from build123d import *

# Parameters (mm, degrees)
F1_W     = 1
F1_H     = 1
F1_W_2   = 13
F2_DEPTH = 0.5


with BuildPart() as f2:
    # F1 (on Top) → F2 (new body)
    with BuildSketch(Plane.XY):
        with BuildLine():
            ThreePointArc((38, -47.5), (37.7071067812, -46.7928932188), (37, -46.5))
            Line((37, -46.5), (37, -47.5))
            Line((37, -47.5), (36, -47.5))
            ThreePointArc((36, -47.5), (36.2928932188, -48.2071067812), (37, -48.5))
            ThreePointArc((37, -48.5), (37.7071067812, -48.2071067812), (38, -47.5))
        make_face()
        with BuildLine():
            Line((36, -46.5), (37, -46.5))
            ThreePointArc((37, -46.5), (37.7071067812, -46.7928932188), (38, -47.5))
            Line((38, -47.5), (38, 47.5))
            ThreePointArc((38, 47.5), (37, 48.5), (36, 47.5))
            Line((36, 47.5), (36, -46.5))
        make_face()
        with Locations((36.5, -47)):
            Rectangle(F1_W, F1_H)
        with Locations((29.5, -47)):
            Rectangle(F1_W_2, F1_H)
        with BuildLine():
            ThreePointArc((37, -48.5), (36.2928932188, -48.2071067812), (36, -47.5))
            Line((36, -47.5), (23, -47.5))
            ThreePointArc((23, -47.5), (22.7071067812, -48.2071067812), (22, -48.5))
            Line((22, -48.5), (37, -48.5))
        make_face()
        with BuildLine():
            Line((22, -46.5), (23, -46.5))
            Line((23, -46.5), (23, 47.5))
            ThreePointArc((23, 47.5), (22.7071067812, 46.7928932188), (22, 46.5))
            Line((22, 46.5), (22, -46.5))
        make_face()
        with Locations((22.5, -47)):
            Rectangle(F1_W, F1_H)
        with BuildLine():
            ThreePointArc((22, -48.5), (22.7071067812, -48.2071067812), (23, -47.5))
            Line((23, -47.5), (22, -47.5))
            Line((22, -47.5), (22, -46.5))
            ThreePointArc((22, -46.5), (21.2928932188, -46.7928932188), (21, -47.5))
            ThreePointArc((21, -47.5), (21.2928932188, -48.2071067812), (22, -48.5))
        make_face()
        with BuildLine():
            ThreePointArc((22, 46.5), (22.7071067812, 46.7928932188), (23, 47.5))
            ThreePointArc((23, 47.5), (22.7071067812, 48.2071067812), (22, 48.5))
            ThreePointArc((22, 48.5), (21.2928932188, 48.2071067812), (21, 47.5))
            Line((21, 47.5), (22, 47.5))
            Line((22, 47.5), (22, 46.5))
        make_face()
        with BuildLine():
            ThreePointArc((21, -47.5), (21.2928932188, -46.7928932188), (22, -46.5))
            Line((22, -46.5), (22, 46.5))
            Line((22, 46.5), (21, 46.5))
            Line((21, 46.5), (21, -47.5))
        make_face()
        with BuildLine():
            ThreePointArc((21, 47.5), (21.2928932188, 48.2071067812), (22, 48.5))
            Line((22, 48.5), (7, 48.5))
            ThreePointArc((7, 48.5), (7.7071067812, 48.2071067812), (8, 47.5))
            Line((8, 47.5), (21, 47.5))
        make_face()
        with Locations((21.5, 47)):
            Rectangle(F1_W, F1_H)
        with Locations((14.5, 47)):
            Rectangle(F1_W_2, F1_H)
        with BuildLine():
            ThreePointArc((8, 47.5), (7.7071067812, 48.2071067812), (7, 48.5))
            ThreePointArc((7, 48.5), (6.2928932188, 48.2071067812), (6, 47.5))
            ThreePointArc((6, 47.5), (6.2928932188, 46.7928932188), (7, 46.5))
            Line((7, 46.5), (7, 47.5))
            Line((7, 47.5), (8, 47.5))
        make_face()
        with BuildLine():
            Line((8, -47.5), (8, 46.5))
            Line((8, 46.5), (7, 46.5))
            Line((7, 46.5), (7, -46.5))
            ThreePointArc((7, -46.5), (7.7071067812, -46.7928932188), (8, -47.5))
        make_face()
        with Locations((7.5, 47)):
            Rectangle(F1_W, F1_H)
        with BuildLine():
            ThreePointArc((7, 46.5), (6.2928932188, 46.7928932188), (6, 47.5))
            Line((6, 47.5), (6, -46.5))
            Line((6, -46.5), (7, -46.5))
            Line((7, -46.5), (7, 46.5))
        make_face()
        with BuildLine():
            ThreePointArc((7, -48.5), (7.7071067812, -48.2071067812), (8, -47.5))
            ThreePointArc((8, -47.5), (7.7071067812, -46.7928932188), (7, -46.5))
            Line((7, -46.5), (7, -47.5))
            Line((7, -47.5), (6, -47.5))
            ThreePointArc((6, -47.5), (6.2928932188, -48.2071067812), (7, -48.5))
        make_face()
        with Locations((6.5, -47)):
            Rectangle(F1_W, F1_H)
        with Locations((-0.5, -47)):
            Rectangle(F1_W_2, F1_H)
        with BuildLine():
            Line((-8, -48.5), (7, -48.5))
            ThreePointArc((7, -48.5), (6.2928932188, -48.2071067812), (6, -47.5))
            Line((6, -47.5), (-7, -47.5))
            ThreePointArc((-7, -47.5), (-7.2928932188, -48.2071067812), (-8, -48.5))
        make_face()
        with Locations((-7.5, -47)):
            Rectangle(F1_W, F1_H)
        with BuildLine():
            Line((-8, -46.5), (-7, -46.5))
            Line((-7, -46.5), (-7, 47.5))
            ThreePointArc((-7, 47.5), (-7.2928932188, 46.7928932188), (-8, 46.5))
            Line((-8, 46.5), (-8, -46.5))
        make_face()
        with BuildLine():
            ThreePointArc((-9, -47.5), (-8.7071067812, -48.2071067812), (-8, -48.5))
            ThreePointArc((-8, -48.5), (-7.2928932188, -48.2071067812), (-7, -47.5))
            Line((-7, -47.5), (-8, -47.5))
            Line((-8, -47.5), (-8, -46.5))
            ThreePointArc((-8, -46.5), (-8.7071067812, -46.7928932188), (-9, -47.5))
        make_face()
        with BuildLine():
            ThreePointArc((-9, -47.5), (-8.7071067812, -46.7928932188), (-8, -46.5))
            Line((-8, -46.5), (-8, 46.5))
            Line((-8, 46.5), (-9, 46.5))
            Line((-9, 46.5), (-9, -47.5))
        make_face()
        with BuildLine():
            ThreePointArc((-8, 46.5), (-7.2928932188, 46.7928932188), (-7, 47.5))
            ThreePointArc((-7, 47.5), (-7.2928932188, 48.2071067812), (-8, 48.5))
            ThreePointArc((-8, 48.5), (-8.7071067812, 48.2071067812), (-9, 47.5))
            Line((-9, 47.5), (-8, 47.5))
            Line((-8, 47.5), (-8, 46.5))
        make_face()
        with Locations((-8.5, 47)):
            Rectangle(F1_W, F1_H)
        with BuildLine():
            ThreePointArc((-9, 47.5), (-8.7071067812, 48.2071067812), (-8, 48.5))
            Line((-8, 48.5), (-23, 48.5))
            ThreePointArc((-23, 48.5), (-22.2928932188, 48.2071067812), (-22, 47.5))
            Line((-22, 47.5), (-9, 47.5))
        make_face()
        with Locations((-15.5, 47)):
            Rectangle(F1_W_2, F1_H)
        with BuildLine():
            ThreePointArc((-22, 47.5), (-22.2928932188, 48.2071067812), (-23, 48.5))
            ThreePointArc((-23, 48.5), (-23.7071067812, 48.2071067812), (-24, 47.5))
            ThreePointArc((-24, 47.5), (-23.7071067812, 46.7928932188), (-23, 46.5))
            Line((-23, 46.5), (-23, 47.5))
            Line((-23, 47.5), (-22, 47.5))
        make_face()
        with Locations((-22.5, 47)):
            Rectangle(F1_W, F1_H)
        with BuildLine():
            Line((-22, -47.5), (-22, 46.5))
            Line((-22, 46.5), (-23, 46.5))
            Line((-23, 46.5), (-23, -46.5))
            ThreePointArc((-23, -46.5), (-22.2928932188, -46.7928932188), (-22, -47.5))
        make_face()
        with BuildLine():
            ThreePointArc((-23, 46.5), (-23.7071067812, 46.7928932188), (-24, 47.5))
            Line((-24, 47.5), (-24, -46.5))
            Line((-24, -46.5), (-23, -46.5))
            Line((-23, -46.5), (-23, 46.5))
        make_face()
        with BuildLine():
            ThreePointArc((-23, -48.5), (-22.2928932188, -48.2071067812), (-22, -47.5))
            ThreePointArc((-22, -47.5), (-22.2928932188, -46.7928932188), (-23, -46.5))
            Line((-23, -46.5), (-23, -47.5))
            Line((-23, -47.5), (-24, -47.5))
            ThreePointArc((-24, -47.5), (-23.7071067812, -48.2071067812), (-23, -48.5))
        make_face()
        with Locations((-30.5, -47)):
            Rectangle(F1_W_2, F1_H)
        with Locations((-23.5, -47)):
            Rectangle(F1_W, F1_H)
        with BuildLine():
            Line((-38, -48.5), (-23, -48.5))
            ThreePointArc((-23, -48.5), (-23.7071067812, -48.2071067812), (-24, -47.5))
            Line((-24, -47.5), (-37, -47.5))
            ThreePointArc((-37, -47.5), (-37.2928932188, -48.2071067812), (-38, -48.5))
        make_face()
        with BuildLine():
            Line((-38, -46.5), (-37, -46.5))
            Line((-37, -46.5), (-37, 47.5))
            ThreePointArc((-37, 47.5), (-38, 48.5), (-39, 47.5))
            Line((-39, 47.5), (-39, -47.5))
            ThreePointArc((-39, -47.5), (-38.7071067812, -46.7928932188), (-38, -46.5))
        make_face()
        with Locations((-37.5, -47)):
            Rectangle(F1_W, F1_H)
        with BuildLine():
            ThreePointArc((-39, -47.5), (-38.7071067812, -48.2071067812), (-38, -48.5))
            ThreePointArc((-38, -48.5), (-37.2928932188, -48.2071067812), (-37, -47.5))
            Line((-37, -47.5), (-38, -47.5))
            Line((-38, -47.5), (-38, -46.5))
            ThreePointArc((-38, -46.5), (-38.7071067812, -46.7928932188), (-39, -47.5))
        make_face()
    extrude(amount=F2_DEPTH)


solid = f2.part
Verification items for the finished model (mm, model axes). Give positions to 0.01 mm unless a question says otherwise; leave off trailing zeros. Write each loop counter-clockwise with the first axis right and the second up, starting at its lowest first coordinate (ties: lowest second). Pieces come first, ordered by that corner, then holes. Notation, with made-up numbers: M 63,-35.75 L 93,-35.75 A11 cw 93,-28.75 Z; hole C 56,25 d9. An arc over 180 degrees is marked long. Put each result on its own line as item: value. Start each with the question number.
1. Section check C-C (x = 15). Record the cut outline in (y, z).
2. Go/stop test with a flat-tipped pin: pin 1 Ø1.5 at (x, y) = (25, -4.5) entering from +Z. Record where the tip stops, or that it passes through.
3. Scan lines: line 1 along X through (y, z) = (27, 0.45); line 2 along Y through (x, z) = (-26, 0.4); line 3 along Y through (x, z) = (18.5, 0.2). Record each from-to range of solid material in increasing order. Write a range as [from, to].
4. Section check A-A (y = -32). Record the cut outline in (x, z), and give its area (3 significant figures).
Answer list:
1. outline: M 46.5,0 L 48.5,0 L 48.5,0.5 L 46.5,0.5 Z
2. pin 1: through
3. line 1: [-39, -37], [-24, -22], [-9, -7], [6, 8], [21, 23], [36, 38]
3. line 2: [-48.5, -46.5]
3. line 3: [46.5, 48.5]
4. outline: M -39,0 L -37,0 L -37,0.5 L -39,0.5 Z; M -24,0 L -22,0 L -22,0.5 L -24,0.5 Z; M -9,0 L -7,0 L -7,0.5 L -9,0.5 Z; M 6,0 L 8,0 L 8,0.5 L 6,0.5 Z; M 21,0 L 23,0 L 23,0.5 L 21,0.5 Z; M 36,0 L 38,0 L 38,0.5 L 36,0.5 Z
4. area: 6.00 mm2
